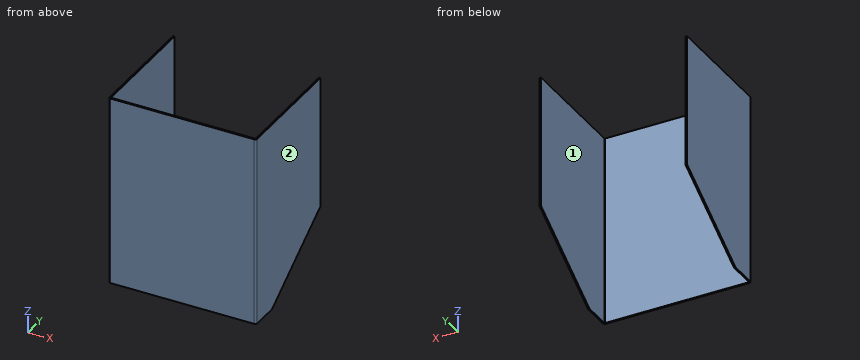
```python
from build123d import *

# Parameters (mm, degrees)
BASE_FLANGE1_DEPTH      = 487
CUT_EXTRUDE1_DEPTH      = 686.604113173
CUT_EXTRUDE1_DEPTH_BACK = 4
CUT_EXTRUDE2_DEPTH      = 686.604113173
CUT_EXTRUDE2_DEPTH_BACK = 4


# Sheet-metal steps are written as plain solids
with BuildPart() as part:
    # Sketch1 → Base-Flange1 (new body)
    with BuildSketch(Plane.XY):
        with BuildLine():
            Line((-185, 300), (-185, 1))
            ThreePointArc((-185, 1), (-184.707106781, 0.292893219), (-184, 0))
            Line((-184, 0), (184, 0))
            ThreePointArc((184, 0), (184.707106781, 0.292893219), (185, 1))
            Line((185, 1), (185, 300))
            Line((185, 300), (189, 300))
            Line((189, 300), (189, 1))
            ThreePointArc((189, 1), (187.535533906, -2.535533906), (184, -4))
            Line((184, -4), (-184, -4))
            ThreePointArc((-184, -4), (-187.535533906, -2.535533906), (-189, 1))
            Line((-189, 1), (-189, 300))
            Line((-189, 300), (-185, 300))
        make_face()
    extrude(amount=BASE_FLANGE1_DEPTH)

    # Sketch7 → Cut-Extrude1 (cut, two sides: drawn at the far end of the back side and taken through both)
    with BuildSketch(Plane(origin=(189, 0, 0), x_dir=(0, 0, -1), z_dir=(1, 0, 0)).offset(-CUT_EXTRUDE1_DEPTH_BACK)):
        Polygon((592.444694682, -839.53580592), (0, 71), (-149, 300), (-741.444694682, 1210.53580592), (1079.626917159, 2395.425195284), (2413.516306522, 345.353583443), align=None)
    extrude(amount=CUT_EXTRUDE1_DEPTH + CUT_EXTRUDE1_DEPTH_BACK, mode=Mode.SUBTRACT)

    # Sketch9 → Cut-Extrude2 (cut, two sides: drawn at the far end of the back side and taken through both)
    with BuildSketch(Plane.ZY.offset(189).offset(-CUT_EXTRUDE2_DEPTH_BACK)):
        Polygon((741.444694682, 1210.53580592), (149, 300), (0, 71), (-592.444694682, -839.53580592), (-2413.516306522, 345.353583443), (-1079.626917159, 2395.425195284), align=None)
    extrude(amount=CUT_EXTRUDE2_DEPTH + CUT_EXTRUDE2_DEPTH_BACK, mode=Mode.SUBTRACT)


solid = part.part
```
Can you work these out from the model? Positions are in its coordinate system, mm. Face numbers are marked on the shaded views. A direction names the side the tool comes from. Coordinates: 2 decimals unless noted, no trailing zeros. Loops run counter-clockwise (first coordinate to the right, second up) from the corner with the lowest first, then second, coordinate; pieces in that order, holes last. Notation, with made-up numbers: (42, 78.25) -> (48, 78.25) arc R12 ccw to (48, 86.25) -> close; hole circle Ø4 at (-17.75, 28). An arc over 180 degrees is marked (long way). Put each result on its own line as item: value. Start each with the question number.
Q1. For the marked faces 1 and 2, which set-ups out of +Z, -Z, +X, -X, +Y, -Y let a thin tool reach every point of the face, with its end or its side?
Q2. I want a section at A-A (y = 280). Write out the boundary of the cut face in (x, z).
Q3. I want a section at C-C (y = 245). Write out the boundary of the cut face in (x, z).
Q4. I want a section at B-B (z = 348). Write out the boundary of the cut face in (x, y).
Q5. If I drill on line 1 (X direction, y = 55.5, z = 88.5); line 2 (Y direction, x = -106, z = 304.5), over which ranges is the centre line in solid material (lowest first)? Write a range as [from, to].
Q6. I'm going to push a flat-ended pin straight in: P1, Ø12, axis at x = -62, z = 62, coming from the +Y side. Where does the tip first touch, or does it pass through?
Q7. I want a section at D-D (x = 22.5). Write out the boundary of the cut face in (y, z), plus the area to 3 significant figures.
Taken from the geometry:
1. face 1: +Z, -Z, +Y
1. face 2: +Z, -Z, +X, +Y, -Y
2. outline: (-189, 135.99) -> (-185, 135.99) -> (-185, 487) -> (-189, 487) -> close; (185, 135.99) -> (189, 135.99) -> (189, 487) -> (185, 487) -> close
3. outline: (-189, 113.21) -> (-185, 113.21) -> (-185, 487) -> (-189, 487) -> close; (185, 113.21) -> (189, 113.21) -> (189, 487) -> (185, 487) -> close
4. outline: (-189, 1) arc R5 ccw to (-184, -4) -> (184, -4) arc R5 ccw to (189, 1) -> (189, 300) -> (185, 300) -> (185, 1) arc R1 cw to (184, 0) -> (-184, 0) arc R1 cw to (-185, 1) -> (-185, 300) -> (-189, 300) -> close
5. line 1: x = [-189, -185], [185, 189]
5. line 2: y = [-4, 0]
6. P1: stops at y = 0
7. outline: (-4, 0) -> (0, 0) -> (0, 487) -> (-4, 487) -> close
7. area: 1,950 mm2
